Geometry check sheet. Reference: drawing and pictorial views, mm from the part's lowest x, y, z. A direction names the side the tool comes from. Coordinates: 2 decimals unless noted, no trailing zeros. Write each loop counter-clockwise with the first axis right and the second up, starting at its lowest first coordinate (ties: lowest second). Pieces come first, ordered by that corner, then holes. Notation, with made-up numbers: (0, -29) -> (28, -29) arc R26 cw to (28, -13) -> close; hole circle Ø5 at (66, 64). An arc over 180 degrees is marked (long way). Use a Markdown table: item, result.
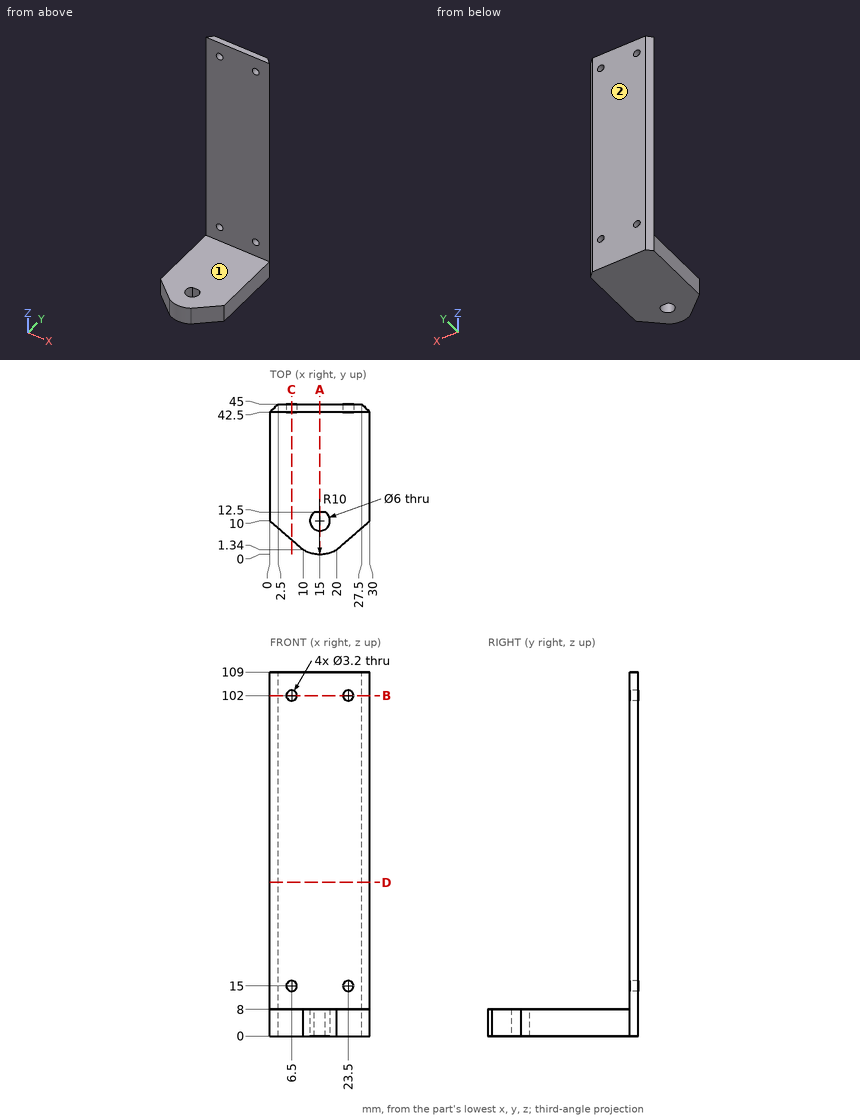
Item 1: Section check D-D on z = 46. Record the boundary of the cut face in (x, y).
Answer block:
| item | result |
|---|---|
| outline | (0, 42.5) -> (30, 42.5) -> (27.5, 45) -> (2.5, 45) -> close |
Item 2: Tool access check on the marked faces 1 and 2. Record the directions out of +Z, -Z, +X, -X, +Y, -Y that give a thin tool (end or side, any length) a straight path to the whole face; none if there is none.
Answer block:
| item | result |
|---|---|
| face 1 | +Z, +X, -X, -Y |
| face 2 | +Z, -Z, +X, -X, +Y |
Item 3: Thickness scan on L1, parallel to Z at x = 23.5, y = 44; L2, parallel to Y at x = 15, z = 1.5; L3, parallel to X at y = 43.1, z = 102. Record the ranges inside material, lowest first. Write a range as [from, to].
Answer block:
| item | result |
|---|---|
| L1 | z = [0, 13.4], [16.6, 100.4], [103.6, 109] |
| L2 | y = [0, 7], [12.5, 45] |
| L3 | x = [0.6, 4.9], [8.1, 21.9], [25.1, 29.4] |
Item 4: Section check A-A on x = 15. Record the boundary of the cut face in (y, z).
Answer block:
| item | result |
|---|---|
| outline | (0, 0) -> (7, 0) -> (7, 8) -> (0, 8) -> close; (12.5, 0) -> (45, 0) -> (45, 109) -> (42.5, 109) -> (42.5, 8) -> (12.5, 8) -> close |
Item 5: Section check B-B on z = 102. Record the boundary of the cut face in (x, y).
Answer block:
| item | result |
|---|---|
| outline | (0, 42.5) -> (4.9, 42.5) -> (4.9, 45) -> (2.5, 45) -> close; (8.1, 42.5) -> (21.9, 42.5) -> (21.9, 45) -> (8.1, 45) -> close; (25.1, 42.5) -> (30, 42.5) -> (27.5, 45) -> (25.1, 45) -> close |
Item 6: Section check C-C on x = 6.5. Record the boundary of the cut face in (y, z).
Answer block:
| item | result |
|---|---|
| outline | (4.37, 0) -> (45, 0) -> (45, 13.4) -> (42.5, 13.4) -> (42.5, 8) -> (4.37, 8) -> close; (42.5, 16.6) -> (45, 16.6) -> (45, 100.4) -> (42.5, 100.4) -> close; (42.5, 103.6) -> (45, 103.6) -> (45, 109) -> (42.5, 109) -> close |
Item 7: Depth check by flat-ended pin: P1, Ø9.5, axis at x = 15, y = 10, coming from the +Z side; P2, Ø1.9, axis at x = 23.5, z = 102, coming from the -Y side; P3, Ø15, axis at x = 9, z = 57, coming from the -Y side; P4, Ø1, axis at x = 14, z = 2.5, coming from the -Y side. Enter the tip coordinate at first touch or a pass-through.
Answer block:
| item | result |
|---|---|
| P1 | stops at z = 8 |
| P2 | passes through |
| P3 | stops at y = 42.5 |
| P4 | stops at y = 0.01 |
